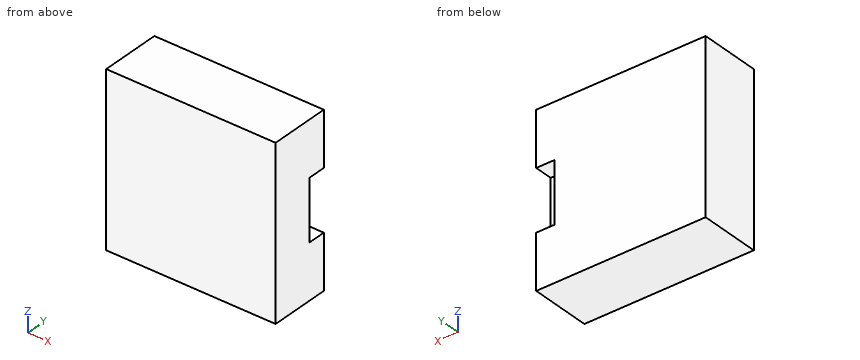
```python
from build123d import *

# Parameters (mm, degrees)
SKETCH1_W           = 28
SKETCH1_H           = 28
BOSS_EXTRUDE1_DEPTH = 5
SKETCH2_W           = 3
SKETCH2_H           = 3
CUT_EXTRUDE1_DEPTH  = 5


with BuildPart() as part:
    # Sketch1 → Boss-Extrude1 (new body, symmetric)
    with BuildSketch(Plane(origin=(0, 0, 0), x_dir=(1, 0, 0), z_dir=(0, 1, 0))):
        Rectangle(SKETCH1_W, SKETCH1_H)
    extrude(amount=BOSS_EXTRUDE1_DEPTH, both=True)

    # Sketch2 → Cut-Extrude1 (cut, symmetric)
    with BuildSketch(Plane.XY):
        with Locations((12.5, 3.5)):
            Rectangle(SKETCH2_W, SKETCH2_H)
    extrude(amount=CUT_EXTRUDE1_DEPTH, both=True, mode=Mode.SUBTRACT)


solid = part.part
```
Could you check a few things on this model? Use its own coordinates, in mm. Coordinates: 2 decimals unless noted, no trailing zeros. Write each loop counter-clockwise with the first axis right and the second up, starting at its lowest first coordinate (ties: lowest second). Pieces come first, ordered by that corner, then holes. Notation, with made-up numbers: (63, 54.5) -> (91, 54.5) arc R7 cw to (91, 64.5) -> close; hole circle Ø4 at (-31, 13). An arc over 180 degrees is marked (long way). Write item = value, one per line. Start each with the question number.
(1) I want a section at A-A (x = 11.5). Please give me the cut outline in (y, z), plus the area to 3 significant figures.
(2) I need wall thicknesses on line 1 (Z direction, x = 12.25, y = 4); line 2 (Y direction, x = 12.5, z = 2); line 3 (X direction, y = 3, z = -2.5). Which ranges of each line are inside material? Lowest first, please. Write a range as [from, to].
(3) I want a section at B-B (z = -2.5). Please give me the cut outline in (x, y), plus the area to 3 significant figures.
(4) Will this pin go through, and if not, where does the flat tip stop? pin 1 (3.5 mm diameter, centred on y = 3, z = 0.5, fed in from +X).
Result set:
q1.outline = (-5, -14) -> (5, -14) -> (5, -5) -> (2, -5) -> (2, 5) -> (5, 5) -> (5, 14) -> (-5, 14) -> close
q1.area = 250 mm2
q2.line_1 = [-14, -5], [5, 14]
q2.line_2 = [-5, 2]
q2.line_3 = [-14, 11]
q3.outline = (-14, -5) -> (14, -5) -> (14, 2) -> (11, 2) -> (11, 5) -> (-14, 5) -> close
q3.area = 271 mm2
q4.pin_1 = 14
